Here's how the part is built. I have some questions about the finished solid (model axes, mm). Give positions to 0.01 mm unless a question says otherwise; leave off trailing zeros. Loops run counter-clockwise (first coordinate to the right, second up) from the corner with the lowest first, then second, coordinate; pieces in that order, holes last. Notation, with made-up numbers: M 32.5,-35 L 69.5,-35 A22 ccw 69.5,-10 Z; hole C 61.5,88.5 d5. An arc over 180 degrees is marked long. Answer as CSV lines item,"result". Start each with the question number.
Item 1: If I drill on line 1 along X through (y, z) = (1, -508); line 2 along X through (y, z) = (0.6, -25.4); line 3 along Z through (x, y) = (482.5, 2.2), over which ranges is the centre line in solid material (lowest first)? Write a range as from..to.
Item 2: I want a section at C-C on x = 232.5. List the corners of the cut face in (y, z) for me, plus the area to 3 significant figures.
Item 3: Will these pins go through, and if not, where does the flat tip stop? P1, Ø8.5, axis at x = 163.51, z = -508, coming from the -Y side; P2, Ø1.3, axis at y = 1, z = -205.5, coming from the -X side.
Item 4: I want a section at B-B on z = -216.5. List the corners of the cut face in (x, y) for me.
Item 5: I want a section at A-A on y = 1.25. Give the number of separate pieces and of enclosed holes in the cut face, plus the area to 3 significant figures.
from build123d import *

# Parameters (mm, degrees)
BOSS_EXTRUDE1_DEPTH = 2.54
SKETCH2_R           = 3.175
CUT_EXTRUDE1_DEPTH  = 3.54


with BuildPart() as part:
    # Sketch1 → Boss-Extrude1 (new body)
    with BuildSketch(Plane(origin=(0, 0, 0), x_dir=(1, 0, 0), z_dir=(0, 1, 0))):
        Polygon((0, 279.4), (0, 546.1), (171.45, 546.1), (171.45, 406.4), (349.25, 406.4), (349.25, 546.1), (520.7, 546.1), (520.7, 279.4), (469.9, 279.4), (469.9, 152.4), (520.7, 152.4), (520.7, 0), (0, 0), (0, 152.4), (50.8, 152.4), (50.8, 279.4), align=None)
    extrude(amount=BOSS_EXTRUDE1_DEPTH)

    # Sketch2 → Cut-Extrude1 (cut, through all)
    with BuildSketch(Plane(origin=(0, 2.54, 0), x_dir=(1, 0, 0), z_dir=(0, 1, 0))):
        with Locations((7.9375, 508)):
            Circle(SKETCH2_R)
        with Locations((163.5125, 508)):
            Circle(SKETCH2_R)
        with Locations((7.9375, 431.8)):
            Circle(SKETCH2_R)
        with Locations((163.5125, 431.8)):
            Circle(SKETCH2_R)
        with Locations((7.9375, 304.8)):
            Circle(SKETCH2_R)
        with Locations((7.9375, 101.6)):
            Circle(SKETCH2_R)
        with Locations((7.9375, 25.4)):
            Circle(SKETCH2_R)
        with Locations((512.7625, 25.4)):
            Circle(SKETCH2_R)
        with Locations((512.7625, 101.6)):
            Circle(SKETCH2_R)
        with Locations((512.7625, 304.8)):
            Circle(SKETCH2_R)
        with Locations((357.1875, 431.8)):
            Circle(SKETCH2_R)
        with Locations((512.7625, 431.8)):
            Circle(SKETCH2_R)
        with Locations((357.1875, 508)):
            Circle(SKETCH2_R)
        with Locations((512.7625, 508)):
            Circle(SKETCH2_R)
    extrude(amount=-CUT_EXTRUDE1_DEPTH, mode=Mode.SUBTRACT)


solid = part.part
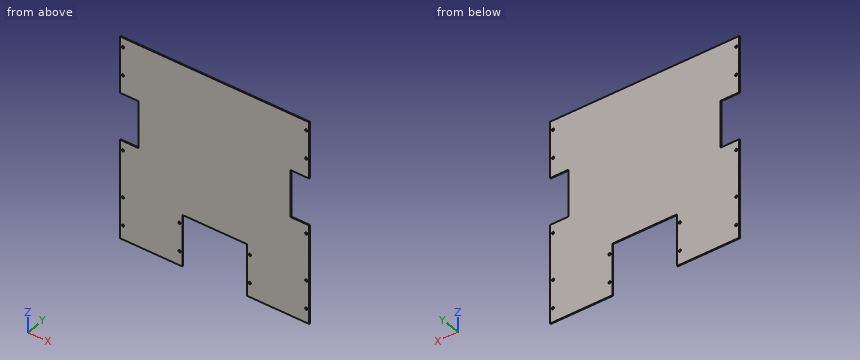
Result:
1,line 1,"0..4.76, 11.11..160.34, 166.69..171.45, 349.25..354.01, 360.36..509.59, 515.94..520.7"
1,line 2,"0..4.76, 11.11..509.59, 515.94..520.7"
1,line 3,"-546.1..-279.4, -152.4..0"
2,outline,"M 0,-406.4 L 2.54,-406.4 L 2.54,0 L 0,0 Z"
2,area,"1,030 mm^2"
3,P1,"y = 0"
3,P2,"x = 50.8"
4,outline,"M 50.8,0 L 469.9,0 L 469.9,2.54 L 50.8,2.54 Z"
5,separate pieces,"1"
5,enclosed holes,"14"
5,area,"246,000 mm^2"
